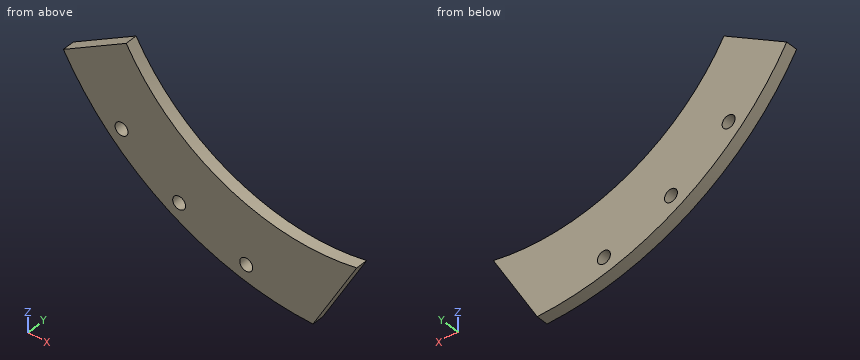
Autodesk Inventor part; units mm, degrees
ref_plane "YZ Plane" through (0, 0, 0) normal (1, 0, 0) x (0, 1, 0)
ref_plane "XZ Plane" through (0, 0, 0) normal (0, 1, 0) x (-1, 0, 0)
ref_plane "XY Plane" through (0, 0, 0) normal (0, 0, 1) x (1, 0, 0)
sketch "スケッチ1" plane through (0, 0, 0) normal (0, 1, 0) x (-1, 0, 0)
  circle A0 centre (0, 0) radius 27.5
  line L0 (13, 12.85) -> (-13, 12.85)
  line L1 (-13, 12.85) -> (-13, -12.85)
  line L2 (-13, -12.85) -> (13, -12.85)
  line L3 (13, -12.85) -> (13, 12.85)
  circle A1 centre (0, 0) radius 32.5 construction
  circle A2 centre (0, 0) radius 36.5
  line L4 (0, 0) -> (18.4986, -32.0406)
  line L5 (0, 0) -> (31.6099, -18.25)
  line L6 (-13, -12.85) -> (0.651, -36.4942)
  line L7 (13.2, 12.8507) -> (13.2, -12.85)
  line L8 (13.2, -12.85) -> (13, -12.85)
  circle A3 centre (0, 0) radius 34.5 construction
  circle A4 centre (24.3952, -24.3952) radius 0.8
  circle A5 centre (8.9293, -33.3244) radius 0.8
  circle A6 centre (17.25, -29.8779) radius 0.8
  line L9 (0, 0) -> (24.3952, -24.3952) construction
  line L10 (0, 0) -> (8.9293, -33.3244) construction
  point P0 (13, 0)
  point P1 (0, 12.85)
  point P2 (13, -34.1065)
  point P3 (-13, -34.1065)
  point P4 (28.1458, -16.25)
  point P5 (13, -7.5056)
  point P6 (18.25, -31.6099)
  point P7 (16.25, -28.1458)
  point P8 (23.8157, -13.75)
  point P9 (-4.7839, -27.0807)
  point P10 (-1.6802, -32.4565)
  point P11 (13.2, -7.621)
  dimension "d0" = 55
  dimension "d1" = 12.85
  dimension "d2" = 26
  dimension "d3" = 5
  dimension "d4" = 4
  dimension "d11" = 60
  dimension "d12" = 30
  dimension "d16" = 0.2
  dimension "d19" = 2
  dimension "d20" = 1.6
  dimension "d21" = 1.6
  dimension "d22" = 1.6
  dimension "d23" = 15
  dimension "d24" = 15
extrude "押し出し4" add sketch "スケッチ1" along normal blind 1.5 contours A0 L4 A6 A2 L6 | L5 A2 L4 A6 A0
equation "\"d23\" = 0.5 * d12"
equation "\"d24\" = d23"
properties part number "waist_side_cover"
The listing builds one solid part. Answer for the finished solid, in the listing's coordinates (mm). Coordinates: 2 decimals unless noted, no trailing zeros. Loops run counter-clockwise (first coordinate to the right, second up) from the corner with the lowest first, then second, coordinate; pieces in that order, holes last. Notation, with made-up numbers: (-3.75, -29.5) -> (49.25, -29.5) arc R9 ccw to (49.25, -25.5) -> close; hole circle Ø1 at (28, -8). An arc over 180 degrees is marked (long way). Answer in a Markdown table with one row per item. Add a question column.
1. The part is cut by section A-A, the plane x = -17.25. Write down the section's boundary in (y, z), then the cut area to 3 significant figures.
2. A flat-ended cylindrical pin translates along its axis: P1, Ø6, axis at x = -27, z = -31, coming from the -Y side. Find the tip coordinate at first contact, or state that the pin passes through.
3. The part is cut by section C-C, the plane y = 0.3. Write down the section's boundary in (x, z), then the cut area to 3 significant figures.
4. The part is cut by section D-D, the plane x = -21.5. Write down the section's boundary in (y, z), then the cut area to 3 significant figures.
5. The part is cut by section B-B, the plane z = -24. Write down the section's boundary in (x, y), then the cut area to 3 significant figures.
6. Consider line 1 (Z direction, x = -17.25, y = 0.8); line 2 (Z direction, x = -24, y = 0.35); line 3 (Z direction, x = -26, y = 0.25). Determine where each line is inside the solid, lowest interval first. Write a range as [from, to].
Answer below:
| question | item | result |
|---|---|---|
| 1 | outline | (0, -32.17) -> (1.5, -32.17) -> (1.5, -30.68) -> (0, -30.68) -> close; (0, -29.08) -> (1.5, -29.08) -> (1.5, -21.42) -> (0, -21.42) -> close |
| 1 | area | 13.7 mm2 |
| 2 | P1 | through |
| 3 | outline | (-31.61, -18.25) arc R36.5 ccw to (-0.65, -36.49) -> (4.78, -27.08) arc R27.5 cw to (-23.82, -13.75) -> close; hole circle Ø1.6 at (-24.4, -24.4); hole circle Ø1.6 at (-17.25, -29.88); hole circle Ø1.6 at (-8.93, -33.32) |
| 3 | area | 314 mm2 |
| 4 | outline | (0, -29.5) -> (1.5, -29.5) -> (1.5, -17.15) -> (0, -17.15) -> close |
| 4 | area | 18.5 mm2 |
| 5 | outline | (-27.5, 0) -> (-25.09, 0) -> (-25.09, 1.5) -> (-27.5, 1.5) -> close; (-23.7, 0) -> (-13.43, 0) -> (-13.43, 1.5) -> (-23.7, 1.5) -> close |
| 5 | area | 19.0 mm2 |
| 6 | line 1 | [-32.17, -30.68], [-29.08, -21.42] |
| 6 | line 2 | [-27.5, -25.09], [-23.7, -13.86] |
| 6 | line 3 | [-25.62, -15.01] |
